```python
from build123d import *

# Parameters (mm, degrees)
ESQUISSE1_W                                   = 45
ESQUISSE1_H                                   = 45
BOSS_EXTRU_1_DEPTH                            = 5
TROU_POUR_TARAUDAGE_POUR_TROU_TARAUD_M3_D     = 2.5
TROU_POUR_TARAUDAGE_POUR_TROU_TARAUD_M3_DEPTH = 10
TROU_POUR_TARAUDAGE_POUR_TROU_TARAUD_M3_TIP   = 0.751075774


with BuildPart() as part:
    # Esquisse1 → Boss.-Extru.1 (new body)
    with BuildSketch(Plane.XY):
        with Locations((22.5, 22.5)):
            Rectangle(ESQUISSE1_W, ESQUISSE1_H)
    extrude(amount=BOSS_EXTRU_1_DEPTH)

    # Trou pour taraudage pour trou taraudé M3x0.51
    with Locations(Plane.XY.offset(5)):
        with Locations((5, 40), (40, 5), (40, 40), (5, 5)):
            Hole(TROU_POUR_TARAUDAGE_POUR_TROU_TARAUD_M3_D / 2, depth=TROU_POUR_TARAUDAGE_POUR_TROU_TARAUD_M3_DEPTH)
            with Locations((0, 0, -(TROU_POUR_TARAUDAGE_POUR_TROU_TARAUD_M3_DEPTH + TROU_POUR_TARAUDAGE_POUR_TROU_TARAUD_M3_TIP / 2))):  # 118° drill point
                Cone(0, TROU_POUR_TARAUDAGE_POUR_TROU_TARAUD_M3_D / 2, TROU_POUR_TARAUDAGE_POUR_TROU_TARAUD_M3_TIP, mode=Mode.SUBTRACT)


solid = part.part
```
Can you work these out from the model? Positions are in its coordinate system, mm. Coordinates: 2 decimals unless noted, no trailing zeros. Loops run counter-clockwise (first coordinate to the right, second up) from the corner with the lowest first, then second, coordinate; pieces in that order, holes last.
Item 1: If we mould it in two halves opening along X, with no side actions, what happens to faces 1 (the face through (5.16, 41.24, 2.46)), 2 (the face through (40.99, 4.24, 2.46)), 3 (the face through (45, 22, 2)), 4 (the face through (22, 0, 2))? For each: released by +X, released by -X, zero draft, split by the parting line, or undercut.
Answers below:
face 1: undercut
face 2: undercut
face 3: released by +X
face 4: zero draft
Item 2: Suppose I cut it at A-A (y = 40). Please give me the cut outline in (x, z).
Answers below:
outline: (0, 0) - (3.75, 0) - (3.75, 5) - (0, 5) - close; (6.25, 0) - (38.75, 0) - (38.75, 5) - (6.25, 5) - close; (41.25, 0) - (45, 0) - (45, 5) - (41.25, 5) - close
Item 3: Please list where these lines run through material, in increasing order: L1, parallel to Y at x = 40, z = 3.7; L2, parallel to X at y = 41, z = 3.7; L3, parallel to X at y = 40.5, z = 4.5.
Answers below:
L1: y = 0 to 3.75, 6.25 to 38.75, 41.25 to 45
L2: x = 0 to 4.25, 5.75 to 39.25, 40.75 to 45
L3: x = 0 to 3.85, 6.15 to 38.85, 41.15 to 45
